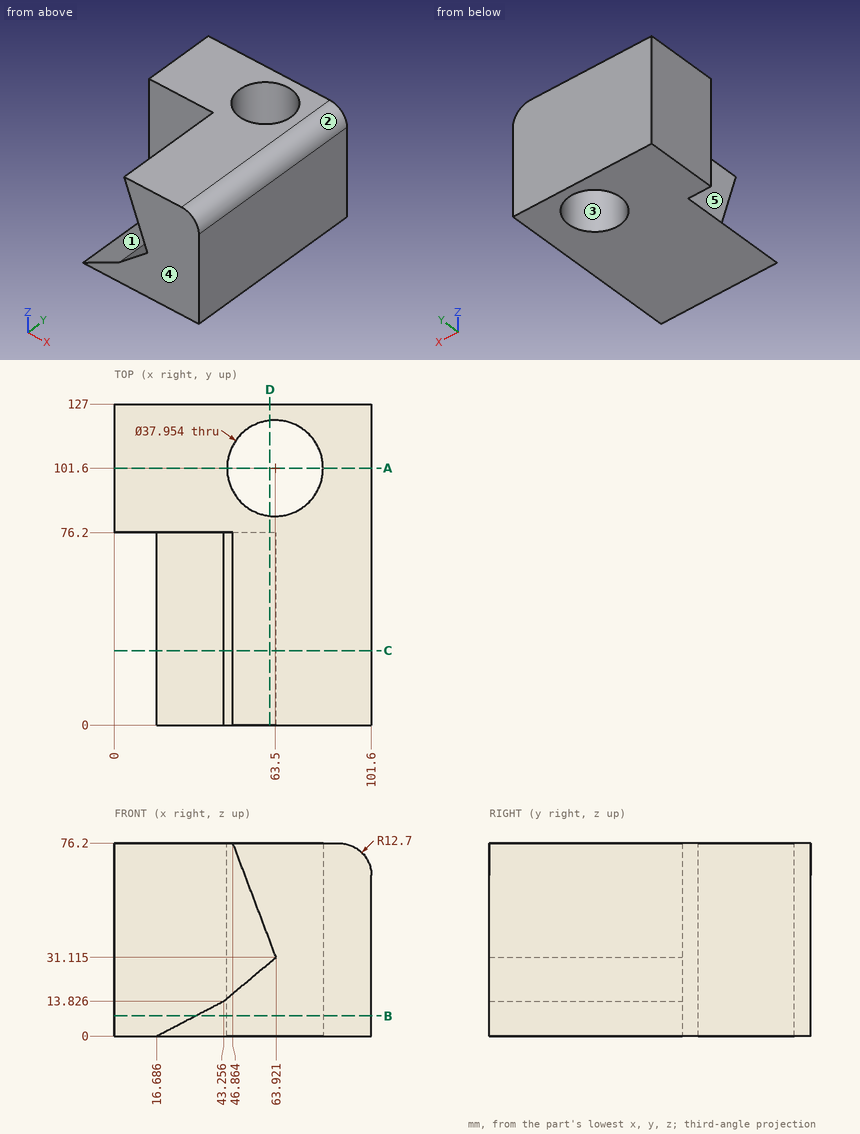
Design review of the part shown in the three views and the two pictorial views. Dimensions are in mm from the part's minimum x, y and z. A direction names the side the tool comes from. Coordinates: 2 decimals unless noted, no trailing zeros. Loops run counter-clockwise (first coordinate to the right, second up) from the corner with the lowest first, then second, coordinate; pieces in that order, holes last. Notation, with made-up numbers: (-27.75, -2) - (-23.75, -2) arc R26 ccw to (-23.75, 27) - close; hole circle Ø6 at (-29, -34). An arc over 180 degrees is marked (long way). Use a Markdown table: item, result. Add a question column.
Item 1: Insertion check: pin 1 Ø3 at (x, z) = (15, 48.5) entering from -Y; pin 2 Ø2 at (y, z) = (19.5, 47.5) entering from -X. Each pin has a flat end and moves straight along its axis. Give the tip position at first contact, or say it passes through.
Item 2: For line 1 (X direction, y = 101, z = 58); line 2 (Y direction, x = 63, z = 32); line 3 (Y direction, x = 63.5, z = 56.5), list the stretches that pass through material, from the lowest coordinate up.
Item 3: Tool access review of the marked faces 1 and 2: name each direction out of +Z, -Z, +X, -X, +Y, -Y from which nothing blocks a thin tool from reaching the whole face with its end or side.
Item 4: We need section D-D (x = 61.5). Give the boundary of the cut face in (y, z), and give its area (3 significant figures).
Item 5: We need section B-B (z = 8). Give the boundary of the cut face in (x, y) (1 decimal), and give its area (3 significant figures).
Item 6: We need section A-A (y = 101.6). Give the boundary of the cut face in (x, z).
Item 7: We need section C-C (y = 29.5). Give the boundary of the cut face in (x, z) (1 decimal).
Item 8: Mouldability with a two-part tool opening along X and no side actions: class the marked faces 3, 4 and 5 as pulls with the +X half, pulls with the -X half, needs draft (parallel to the pull), parting line crosses it, or undercut.
Results list:
| question | item | result |
|---|---|---|
| 1 | pin 1 | stops at y = 76.2 |
| 1 | pin 2 | stops at x = 57.34 |
| 2 | line 1 | x = 0 to 44.53, 82.47 to 101.6 |
| 2 | line 2 | y = 76.2 to 82.63, 120.57 to 127 |
| 2 | line 3 | y = 0 to 82.62, 120.58 to 127 |
| 3 | face 1 | +Z, -X, -Y |
| 3 | face 2 | +Z, +X, +Y, -Y |
| 4 | outline | (0, 0) - (82.73, 0) - (82.73, 76.2) - (0, 76.2) - (0, 37.51) - (76.2, 37.51) - (76.2, 29.09) - (0, 29.09) - close; (120.47, 0) - (127, 0) - (127, 76.2) - (120.47, 76.2) - close |
| 4 | area | 6,160 mm^2 |
| 5 | outline | (0, 76.2) - (32.1, 76.2) - (32.1, 0) - (101.6, 0) - (101.6, 127) - (0, 127) - close; hole circle Ø38 at (63.5, 101.6) |
| 5 | area | 9,330 mm^2 |
| 6 | outline | (0, 0) - (44.52, 0) - (44.52, 76.2) - (0, 76.2) - close; (82.48, 0) - (101.6, 0) - (101.6, 63.5) arc R12.7 ccw to (88.9, 76.2) - (82.48, 76.2) - close |
| 7 | outline | (16.7, 0) - (101.6, 0) - (101.6, 63.5) arc R12.7 ccw to (88.9, 76.2) - (46.9, 76.2) - (63.9, 31.1) - (43.3, 13.8) - close |
| 8 | face 3 | undercut |
| 8 | face 4 | needs draft |
| 8 | face 5 | pulls with the -X half |
